```python
from build123d import *

# Parameters (mm, degrees)
F0_R     = 2
F0_R_2   = 5
F0_R_3   = 12
F1_DEPTH = 10
F2_R     = 24.99999
F3_R     = 10
F4_R     = 20


# Not quite as in the source:
# - a fillet or chamfer is up to 0.001 mm smaller than in the source, because OpenCascade refuses the exact size


with BuildPart() as f1:
    # F0 (on Top) → F1 (new body)
    with BuildSketch(Plane.XY):
        Polygon((-26.9614594782, 50), (-66.9614594782, 50), (-66.9614594782, 0), (-26.9614594782, 0), (26.0385405218, -35), (48.0385405218, -35), (48.0385405218, 0), align=None)
        with Locations((28.0385405218, -14)):
            Circle(F0_R, mode=Mode.SUBTRACT)
        with Locations((34.0385405218, -24)):
            Circle(F0_R_2, mode=Mode.SUBTRACT)
        with Locations((40.0385405218, -14)):
            Circle(F0_R, mode=Mode.SUBTRACT)
        with Locations((-41.9614594782, 25)):
            Circle(F0_R_3, mode=Mode.SUBTRACT)
    extrude(amount=F1_DEPTH)

    # F2 (radius 25 in the source; OpenCascade refuses exactly that, so slightly less here)
    f2_edges = [f1.edges().sort_by_distance(p)[0] for p in [
        (-66.961459, 50, 5),
        (-66.961459, 0, 5),
    ]]
    fillet(f2_edges, radius=F2_R)

    # F3
    f3_edges = [f1.edges().sort_by_distance(p)[0] for p in [
        (48.038541, -35, 5),
        (48.038541, 0, 5),
    ]]
    fillet(f3_edges, radius=F3_R)

    # F4
    f4_edges = [f1.edges().sort_by_distance(p)[0] for p in [
        (-26.961459, 50, 5),
        (-26.961459, 0, 5),
        (26.038541, -35, 5),
    ]]
    fillet(f4_edges, radius=F4_R)


solid = f1.part
```
Source: CAD feature listing. Evaluate the final solid. Frame: model axes, mm. A direction names the side the tool comes from. Coordinates: 2 decimals unless noted, no trailing zeros. Order: outer loops, then holes, each group sorted by start corner. A loop starts at its lowest first (then second) coordinate and runs counter-clockwise, first axis right, second up. Notation, with made-up numbers: (-23.5, 86.25) - (31.5, 86.25) arc R16 cw to (31.5, 112.25) - close; hole circle Ø6 at (87.25, -9). An arc over 180 degrees is marked (long way). One line per item, written item: value.
1) Mould query, pull axis X, two halves, no side actions, for faces 3 (the face through (-30.88, 20.4, 4.93)), 4 (the face through (-37, 50, 5)), 5 (the face through (26.371, -34.178, 5.07)), 6 (the face through (11.29, 24.5, 4.93)). Classes: released by +X, released by -X, zero draft, split by the parting line, or undercut.
Computed values:
face 3: undercut
face 4: zero draft
face 5: released by -X
face 6: released by +X
2) Ray query, line 1 (X direction, y = 18.5, z = 8.75); line 2 (Y direction, x = 36.5, z = 6); line 3 (X direction, y = 18, z = 4). Return the intervals inside material, ascending. Write a range as [from, to].
Computed values:
line 1: x = [-66.1, -52.05], [-31.87, 20.29]
line 2: y = [-35, -28.35], [-19.65, 7.69]
line 3: x = [-65.96, -51.71], [-32.21, 21.04]
3) Cut plane C-C on y = -14. Output: boundary loops of the cut face in (x, z).
Computed values:
outline: (-5.76, 0) - (26.04, 0) - (26.04, 10) - (-5.76, 10) - close; (30.04, 0) - (38.04, 0) - (38.04, 10) - (30.04, 10) - close; (42.04, 0) - (48.04, 0) - (48.04, 10) - (42.04, 10) - close
4) Reachability of faces 1 (the face through (30.07, -27.04, 4.93)), 2 (the face through (-38, 0, 5)) from +Z, -Z, +X, -X, +Y, -Y: full face, straight path, thin tool, end or side. Return the list, or none.
Computed values:
face 1: +Z, -Z
face 2: +Z, -Z, -X, -Y
5) Cut plane A-A on z = 4.25. State how many separate pieces and enclosed holes the cut face has, plus the area to 3 significant figures.
Computed values:
separate pieces: 1
enclosed holes: 4
area: 4,720 mm^2
6) Cut plane D-D on y = 21. Output: boundary loops of the cut face in (x, z).
Computed values:
outline: (-66.64, 0) - (-53.28, 0) - (-53.28, 10) - (-66.64, 10) - close; (-30.65, 0) - (16.54, 0) - (16.54, 10) - (-30.65, 10) - close
7) Cut plane B-B on x = -45. Output: boundary loops of the cut face in (y, z).
Computed values:
outline: (0.19, 0) - (13.39, 0) - (13.39, 10) - (0.19, 10) - close; (36.61, 0) - (49.81, 0) - (49.81, 10) - (36.61, 10) - close
8) Contact query for flat-ended pins moving along their axis: pin 1 (4.5 mm diameter, centred on x = -36.5, z = 5.5, fed in from -Y); pin 2 (6 mm diameter, centred on x = -12, z = 3.5, fed in from +Y). Output: stop coordinate, or through.
Computed values:
pin 1: stops at y = 0
pin 2: stops at y = 42.03
